```python
from build123d import *

# Parameters (mm, degrees)
CYLINDER001_R      = 2.5
CYLINDER001_DEPTH  = 10
CYLINDER_R         = 1.25
CYLINDER_DEPTH     = 2
CYLINDER003_R      = 3.5
CYLINDER003_DEPTH  = 20
CYLINDER002_R      = 2
CYLINDER002_DEPTH  = 5
FUSION_PITCH_ANGLE = -90
BOX002_W           = 12
BOX002_H           = 10
BOX002_DEPTH       = 20
BOX001_W           = 10
BOX001_H           = 30
BOX001_DEPTH       = 20
BOX_W              = 12
BOX_H              = 30
BOX_DEPTH          = 30


with BuildPart() as cylinder001:
    # Cylinder001 → Cylinder001 (new body)
    with BuildSketch(Plane(origin=(0, -3, 2), x_dir=(1, 0, 0), z_dir=(0, 0, 1))):
        Circle(CYLINDER001_R)
    extrude(amount=CYLINDER001_DEPTH)


with BuildPart() as fusion002:
    # Cylinder → Cylinder (new body)
    with BuildSketch(Plane(origin=(0, -3, 0), x_dir=(1, 0, 0), z_dir=(0, 0, 1))):
        Circle(CYLINDER_R)
    extrude(amount=CYLINDER_DEPTH)

    # Fusion002: union Cylinder001
    add(cylinder001.part)


with BuildPart() as fusion002_1:
    # Fusion002 placement: moved
    add(fusion002.part.moved(Location((0, -2, 0))))


with BuildPart() as cylinder003:
    # Cylinder003 → Cylinder003 (new body)
    with BuildSketch(Plane(origin=(15, -5, -17), x_dir=(1, 0, 0), z_dir=(0, 0, 1))):
        Circle(CYLINDER003_R)
    extrude(amount=CYLINDER003_DEPTH)


with BuildPart() as cone:
    # Cone → Cone (revolve)
    with BuildSketch(Plane(origin=(15, -5, 5), x_dir=(1, 0, 0), z_dir=(0, 1, 0))):
        Polygon((0, 0), (2, 0), (3.5, 2), (0, 2), align=None)
    revolve(axis=Axis((15, -5, 5), (0, 0, -1)))


with BuildPart() as fusion003:
    # Cylinder002 → Cylinder002 (new body)
    with BuildSketch(Plane(origin=(15, -5, 5), x_dir=(1, 0, 0), z_dir=(0, 0, 1))):
        Circle(CYLINDER002_R)
    extrude(amount=CYLINDER002_DEPTH)

    # Fusion: union Cylinder003, Cone
    add(cylinder003.part)
    add(cone.part)


with BuildPart() as fusion003_1:
    # Fusion pitch: moved
    add(fusion003.part.rotate(Axis((0, 0, 0), (0, 1, 0)), FUSION_PITCH_ANGLE))


with BuildPart() as fusion003_2:
    # Fusion placement: moved
    add(fusion003_1.part.moved(Location((4, 15, 0))))

    # Fusion003: union Fusion002
    add(fusion002_1.part)


with BuildPart() as cube002:
    # Box002 → Box002 (new body)
    with BuildSketch(Plane(origin=(-6, -10, 10), x_dir=(1, 0, 0), z_dir=(0, 0, 1))):
        with Locations((6, 5)):
            Rectangle(BOX002_W, BOX002_H)
    extrude(amount=BOX002_DEPTH)


with BuildPart() as cube001:
    # Box001 → Box001 (new body)
    with BuildSketch(Plane(origin=(6, -10, -10), x_dir=(1, 0, 0), z_dir=(0, 0, 1))):
        with Locations((5, 15)):
            Rectangle(BOX001_W, BOX001_H)
    extrude(amount=BOX001_DEPTH)


with BuildPart() as cut001:
    # Box → Box (new body)
    with BuildSketch(Plane(origin=(-6, -10, 0), x_dir=(1, 0, 0), z_dir=(0, 0, 1))):
        with Locations((6, 15)):
            Rectangle(BOX_W, BOX_H)
    extrude(amount=BOX_DEPTH)

    # Fusion001: union Cube001
    add(cube001.part)

    # Cut: cut Cube002
    add(cube002.part, mode=Mode.SUBTRACT)

    # Cut001: cut Fusion003
    add(fusion003_2.part, mode=Mode.SUBTRACT)


solid = cut001.part
```
Part model, mm, in its own coordinate system. A direction names the side the tool comes from. Round coordinates to 2 decimals unless told otherwise and drop trailing zeros. Loops run counter-clockwise (first coordinate to the right, second up) from the corner with the lowest first, then second, coordinate; pieces in that order, holes last.
Item 1: Drill centre lines: line 1 (Y direction, x = 0, z = 1.2); line 2 (Y direction, x = 3.2, z = 15); line 3 (Y direction, x = -3.5, z = 19). Where is each one in solid material? Low to high.
Item 2: Cut at A-A, the plane x = 0. Give the cut face in (y, z), then the cut area to 3 significant figures.
Item 3: Cut at C-C, the plane z = 15. Give the cut face in (x, y), then the cut area to 3 significant figures.
Item 4: Cut at D-D, the plane x = -3.5. Give the cut face in (y, z).
Item 5: Cut at B-B, the plane y = 10. Give the cut face in (x, z).
Item 6: Mould opens along Z. For faces 5 (the face through (-0.875, 12.044, 14.546)), 6 (the face through (-3.465, 11.352, 13.526)), 7 (the face through (0, 10, 30)), 8 (the face through (6, 10, 20)) say: +Z half, -Z half, draft (parallel to the pull), parting line (faces both ways), or undercut.
Item 7: 3-axis set-ups, long thin cutter, end or side, ignore diameter. For faces 1 (the face through (6, 5, -5)), 2 (the face through (3.535, 6.895, 16.615)), 3 (the face through (-1, -6, 2)), 4 (the face through (0, 0, 20)): which of +Z, -Z, +X, -X, +Y, -Y reach the whole face in a straight line?
Item 8: Drop flat-ended pins along their axis: P1, Ø3, axis at y = 2.5, z = -4.5, coming from the -X side; P2, Ø3, axis at x = 0, y = -5, coming from the +Z side; P3, Ø8, axis at x = 0, y = -5, coming from the +Z side; P4, Ø11, axis at x = 6.5, y = 7.5, coming from the +Z side. Give the stop position or say it passes through.
A:
1. line 1: y = -10 to -6.25, -3.75 to 20
1. line 2: y = 0 to 6.5, 13.5 to 20
1. line 3: y = 0 to 20
2. outline: (-10, 0) - (-6.25, 0) - (-6.25, 2) - (-7.5, 2) - (-7.5, 10) - (-10, 10) - close; (-3.75, 0) - (20, 0) - (20, 30) - (0, 30) - (0, 10) - (-2.5, 10) - (-2.5, 2) - (-3.75, 2) - close; hole circle Ø5.5 at (10, 15)
2. area: 631 mm2
3. outline: (-6, 0) - (6, 0) - (6, 6.5) - (1, 6.5) - (-1, 8) - (-6, 8) - close; (-6, 12) - (-1, 12) - (1, 13.5) - (6, 13.5) - (6, 20) - (-6, 20) - close
3. area: 174 mm2
4. outline: (-10, 0) - (20, 0) - (20, 30) - (0, 30) - (0, 10) - (-10, 10) - close; hole circle Ø4 at (10, 15)
5. outline: (-6, 0) - (6, 0) - (6, -10) - (16, -10) - (16, 10) - (6, 10) - (6, 11.5) - (1, 11.5) - (-1, 13) - (-6, 13) - close; (-6, 17) - (-1, 17) - (1, 18.5) - (6, 18.5) - (6, 30) - (-6, 30) - close
6. face 5: undercut
6. face 6: undercut
6. face 7: +Z half
6. face 8: draft
7. face 1: -Z, -X, +Y, -Y
7. face 2: +X
7. face 3: +Z
7. face 4: +Z, +X, -X, -Y
8. P1: stops at x = 6
8. P2: stops at z = 2
8. P3: stops at z = 10
8. P4: stops at z = 30
